Solid Edge part; units mm, degrees
sketch "Sketch1" plane through (0, 0, 0) normal (0, 0, 1) x (1, 0, 0)
  line L0 (-15, -43.85) -> (-15, 16.15)
  line L1 (-15, 16.15) -> (15, 16.15)
  line L2 (15, 16.15) -> (15, -43.85)
  line L3 (15, -43.85) -> (-15, -43.85)
extrude "Protrusion1" add sketch "Sketch1" against normal blind 7
sketch "Sketch2" plane through (0, 0, 0) normal (0, 0, 1) x (1, 0, 0)
  line L0 (8.25, -14.75) -> (-8.25, -14.75)
  line L1 (-8.25, -14.75) -> (-8.25, 14.75)
  line L2 (-8.25, 14.75) -> (8.25, 14.75)
  line L3 (8.25, 14.75) -> (8.25, -14.75)
extrude "ExtrudedCutout_1" cut sketch "Sketch2" against normal blind 3.9
sketch "Sketch3" plane through (0, -13.85, 0) normal (0, 0, 1) x (1, 0, 0)
  line L0 (3.25, 4.1) -> (-3.25, 4.1)
  line L1 (-3.25, 4.1) -> (-3.25, 5.1)
  line L2 (-3.25, 5.1) -> (-8.25, 5.1)
  line L3 (-8.25, 5.1) -> (-8.25, 17.6)
  line L4 (-3.25, 17.6) -> (-8.25, 17.6)
  line L5 (-3.25, 17.6) -> (-3.25, 23.6)
  line L6 (-3.25, 23.6) -> (3.25, 23.6)
  line L7 (3.25, 23.6) -> (3.25, 4.1)
extrude "Cutout1" cut sketch "Sketch3" against normal up to next
sketch "Sketch4" plane through (0, -13.85, 0) normal (0, 0, 1) x (1, 0, 0)
  line L0 (4.5, 31.4) -> (-4.5, 31.4)
  line L1 (-4.5, 31.4) -> (-4.5, 28.6)
  line L2 (-4.5, 28.6) -> (4.5, 28.6)
  line L3 (4.5, 28.6) -> (4.5, 31.4)
extrude "Cutout2" cut sketch "Sketch4" against normal up to vertex (3.9 mm away)
sketch "Sketch5" plane through (0, -13.85, 0) normal (0, 0, 1) x (1, 0, 0)
  line L0 (7, -4.1577) -> (7, -30)
  line L1 (7, -30) -> (-7, -30)
  line L2 (-7, -30) -> (-7, -4.1577)
  line L3 (-7, -4.1577) -> (-7, -0.9)
  line L4 (-7, -0.9) -> (7, -0.9)
  line L5 (7, -0.9) -> (7, -4.1577)
extrude "Cutout3" cut sketch "Sketch5" against normal up to vertex (3.9 mm away)
sketch "Sketch6" plane through (0, -43.85, -3.5) normal (0, -1, 0) x (1, 0, 0)
  line L0 (-6.2431, 1.55) -> (-7, 1.55)
  line L1 (-7, 1.55) -> (-7, -0.4)
  line L2 (-7, -0.4) -> (7, -0.4)
  line L3 (7, -0.4) -> (7, 1.55)
  line L4 (6.2431, 1.55) -> (7, 1.55)
  line L5 (3.3715, 1.55) -> (5.2431, 1.55)
  line L6 (0.5, 1.55) -> (2.3715, 1.55)
  line L7 (-2.3715, 1.55) -> (-0.5, 1.55)
  line L8 (-5.2431, 1.55) -> (-3.3715, 1.55)
  arc A0 (6.2431, 1.55) -> (5.2431, 1.55) centre (5.7431, 1.55) cw
  arc A1 (3.3715, 1.55) -> (2.3715, 1.55) centre (2.8715, 1.55) cw
  arc A2 (0.5, 1.55) -> (-0.5, 1.55) centre (0, 1.55) cw
  arc A3 (-2.3715, 1.55) -> (-3.3715, 1.55) centre (-2.8715, 1.55) cw
  arc A4 (-5.2431, 1.55) -> (-6.2431, 1.55) centre (-5.7431, 1.55) cw
extrude "ExtrudedProtrusion_2" add sketch "Sketch6" against normal blind 10
sketch "Sketch7" plane through (-8.9522, -13.85, 0) normal (0, 0, 1) x (0, 1, 0)
  circle A0 centre (-25, 2.5478) radius 1.9
  circle A1 centre (-25, -20.4522) radius 1.9
  circle A2 centre (25, 2.5478) radius 1.9
  circle A3 centre (25, -20.4522) radius 1.9
extrude "Cutout4" cut sketch "Sketch7" against normal up to next
sketch "Sketch8" plane through (9.75, -13.85, 0) normal (0, 0, 1) x (0, 1, 0)
  line L0 (-15, 24.75) -> (-15, -5.25)
  line L1 (-15, -5.25) -> (-30, -5.25)
  line L2 (-30, -5.25) -> (-30, 24.75)
  line L3 (-30, 24.75) -> (-15, 24.75)
extrude "Cutout5" cut sketch "Sketch8" against normal up to vertex (1.95 mm away)
fillet "Round_1" radius 2 2 edges at (-11, -28.85, 0) (11, -28.85, 0)
The model under review builds one solid part; all positions refer to its coordinate system, in mm. A direction names the side the tool comes from. Round coordinates to 2 decimals unless told otherwise and drop trailing zeros. Loops run counter-clockwise (first coordinate to the right, second up) from the corner with the lowest first, then second, coordinate; pieces in that order, holes last. Notation, with made-up numbers: (-1, 73) -> (40, 73) arc R33 ccw to (40, 111) -> close; hole circle Ø6 at (66.25, 66.25). An arc over 180 degrees is marked (long way). Return JSON: item names as keys, results as strings.
(1) For line 1 (Y direction, x = -11.5, z = -3.5); line 2 (X direction, y = -38.85, z = -4.9); line 3 (X direction, y = 11.15, z = -3.5), list the stretches that pass through material, from the lowest coordinate up.
Solved:
{"line 1": "-43.85 to -40.75, -36.95 to 9.25, 13.05 to 16.15", "line 2": "-15 to -13.4, -9.6 to 9.6, 13.4 to 15", "line 3": "-15 to -13.4, -9.6 to -8.25, 8.25 to 9.6, 13.4 to 15"}
(2) Add section A-A on y = 11.15. Write out the cut boundary in (x, z).
Solved:
{"outline": "(-15, -7) -> (-13.4, -7) -> (-13.4, 0) -> (-15, 0) -> close; (-9.6, -7) -> (9.6, -7) -> (9.6, 0) -> (8.25, 0) -> (8.25, -3.9) -> (-8.25, -3.9) -> (-8.25, 0) -> (-9.6, 0) -> close; (13.4, -7) -> (15, -7) -> (15, 0) -> (13.4, 0) -> close"}
(3) Add section C-C on z = -3.25. Write out the cut boundary in (x, y).
Solved:
{"outline": "(-15, -43.85) -> (15, -43.85) -> (15, 16.15) -> (4.5, 16.15) -> (4.5, 14.75) -> (8.25, 14.75) -> (8.25, -14.75) -> (7, -14.75) -> (7, -33.85) -> (-7, -33.85) -> (-7, -14.75) -> (-8.25, -14.75) -> (-8.25, 14.75) -> (-4.5, 14.75) -> (-4.5, 16.15) -> (-15, 16.15) -> close; hole circle Ø3.8 at (-11.5, -38.85); hole circle Ø3.8 at (-11.5, 11.15); hole circle Ø3.8 at (11.5, -38.85); hole circle Ø3.8 at (11.5, 11.15)"}
(4) For faces 4 (the flat face through (-8, -14.75, -2)), 5 (the flat face through (-4, -39, -1.95)), 6 (the flat face through (0, -9.75, -5)), list the 3-axis set-ups (+Z, -Z, +X, -X, +Y, -Y) from which the entire face can be reached by the end or side of a thin tool; tool diameter is ignored.
Solved:
{"face 4": "+Z", "face 5": "+Z, +X, -X, -Y", "face 6": "+Z, -Z"}
(5) Add section B-B on x = 11.5. Write out the cut boundary in (y, z).
Solved:
{"outline": "(-43.85, -7) -> (-40.75, -7) -> (-40.75, -1.95) -> (-43.85, -1.95) -> close; (-36.95, -7) -> (9.25, -7) -> (9.25, 0) -> (-26.85, 0) arc R2 ccw to (-28.85, -1.95) -> (-36.95, -1.95) -> close; (13.05, -7) -> (16.15, -7) -> (16.15, 0) -> (13.05, 0) -> close"}
(6) Add section D-D on y = -7. Write out the cut boundary in (x, z).
Solved:
{"outline": "(-15, -7) -> (-8.25, -7) -> (-8.25, 0) -> (-15, 0) -> close; (3.25, -7) -> (15, -7) -> (15, 0) -> (8.25, 0) -> (8.25, -3.9) -> (3.25, -3.9) -> close"}
(7) For pin 1 (0.6 mm diameter, centred on x = -1, z = -2.5, fed in from +Y); pin 2 (4.5 mm diameter, centred on x = 10, y = -38.5, fed in from +Z); pin 3 (3 mm diameter, centred on x = -11.5, y = -38.85, fed in from +Z); pin 4 (5 mm diameter, centred on x = 2.5, y = -8.5, fed in from +Z), all flat-tipped, find the tip position at first contact; note any pin that passes through.
Solved:
{"pin 1": "y = -33.85", "pin 2": "z = -1.95", "pin 3": "through", "pin 4": "z = -3.9"}
(8) The part is to be moulded in two halves that separate along Y. For faces 1 (the flat face through (1, -39, -1.95)), 2 (the flat face through (-7, -22, -2)), 3 (the flat face through (0, -43.85, -4)), say which applies: released by +Y, released by -Y, zero draft, split by the parting line, or undercut.
Solved:
{"face 1": "zero draft", "face 2": "undercut", "face 3": "released by -Y"}
